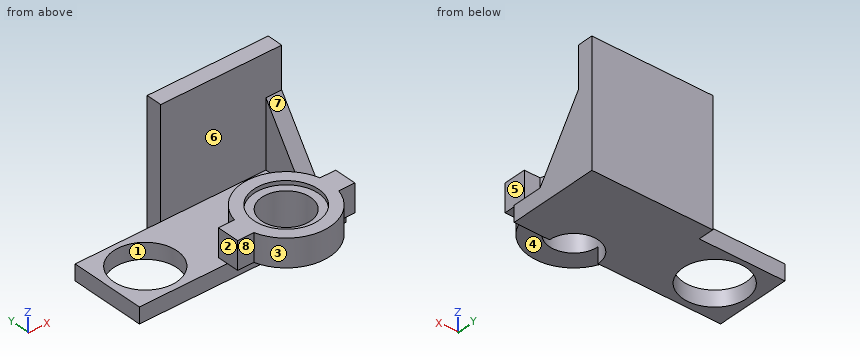
```python
from build123d import *

# Parameters (mm, degrees)
F0_W      = 52.233020775
F0_H      = 18.9497452229
F1_DEPTH  = 4
F2_D      = 16
F4_DEPTH  = 7
F5_R      = 6.15
F6_DEPTH  = 10
F7_R      = 8.15
F8_DEPTH  = 3.72
F9_W      = 30.5920690298
F9_H      = 31.4969494939
F10_DEPTH = 4
F12_DEPTH = 4


with BuildPart() as f1:
    # F0 (on Top) → F1 (new body)
    with BuildSketch(Plane.XY):
        with Locations((-11.0083804466, 9.4748726115)):
            Rectangle(F0_W, F0_H)
    extrude(amount=F1_DEPTH)

    # F2 (through all)
    with Locations(Plane(origin=(0, 0, 0), x_dir=(1, 0, 0), z_dir=(0, 0, -1))):
        with Locations((-27.3946430534, -9.6157854423)):
            Hole(F2_D / 2)

    # F3 (on face) → F4 (join)
    with BuildSketch(Plane.XY.offset(4)):
        with BuildLine():
            Line((-10.8105310121, 2.6503070258), (-14.8572139442, 2.6503070258))
            Line((-14.8572139442, 2.6503070258), (-14.8572139442, -3.0028291512))
            Line((-14.8572139442, -3.0028291512), (-10.7179627347, -3.0028291512))
            ThreePointArc((-10.7179627347, -3.0028291512), (-11.1291732807, -0.1822366147), (-10.8105310121, 2.6503070258))
        make_face()
        with BuildLine():
            ThreePointArc((10.8105310121, 2.6503070258), (0, 11.1306652135), (-10.8105310121, 2.6503070258))
            ThreePointArc((-10.8105310121, 2.6503070258), (-11.1291732807, -0.1822366147), (-10.7179627347, -3.0028291512))
            ThreePointArc((-10.7179627347, -3.0028291512), (0, -11.1306652135), (10.7179627347, -3.0028291512))
            ThreePointArc((10.7179627347, -3.0028291512), (11.1291732807, -0.1822366147), (10.8105310121, 2.6503070258))
        make_face()
        with BuildLine():
            Line((14.7918676957, 2.6503070258), (10.8105310121, 2.6503070258))
            ThreePointArc((10.8105310121, 2.6503070258), (11.1291732807, -0.1822366147), (10.7179627347, -3.0028291512))
            Line((10.7179627347, -3.0028291512), (14.7918676957, -3.0028291512))
            Line((14.7918676957, -3.0028291512), (14.7918676957, 2.6503070258))
        make_face()
    extrude(amount=F4_DEPTH)

    # F5 (on Top) → F6 (cut)
    with BuildSketch(Plane.XY):
        Circle(F5_R)
    extrude(amount=F6_DEPTH, mode=Mode.SUBTRACT)

    # F7 (on face) → F8 (cut)
    with BuildSketch(Plane(origin=(0, 0, 10), x_dir=(1, 0, 0), z_dir=(0, 0, -1))):
        Circle(F7_R)
    extrude(amount=-F8_DEPTH, mode=Mode.SUBTRACT)

    # F9 (on face) → F10 (join)
    with BuildSketch(Plane(origin=(0, 18.9497452229, 0), x_dir=(-1, 0, 0), z_dir=(0, 1, 0))):
        with Locations((0.187904574, 15.7484747469)):
            Rectangle(F9_W, F9_H)
    extrude(amount=F10_DEPTH)

    # F11 (on face) → F12 (join)
    with BuildSketch(Plane.YZ.offset(15.1081299409)):
        Polygon((18.9497452229, 20.9649894387), (7.6817818917, 4), (18.9497452229, 4), align=None)
    extrude(amount=-F12_DEPTH)


solid = f1.part
```
For this review, take the finished solid that the model builds, in its own axes (mm). Face numbers are marked on the shaded views. A direction names the side the tool comes from. Coordinates: 2 decimals unless noted, no trailing zeros. Write each loop counter-clockwise with the first axis right and the second up, starting at its lowest first coordinate (ties: lowest second). Pieces come first, ordered by that corner, then holes. Notation, with made-up numbers: (83, -30.75) -> (132, -30.75) arc R11 cw to (132, -22.75) -> close; hole circle Ø3 at (32.5, -8.5). An arc over 180 degrees is marked (long way). Put each result on its own line as item: value.
Q1. Take a section at A-A, the plane x = 0. State the section outline as (y, z) points, then the cut area to 3 significant figures.
From the geometry:
outline: (-11.13, 4) -> (-6.15, 4) -> (-6.15, 10) -> (-8.15, 10) -> (-8.15, 11) -> (-11.13, 11) -> close; (6.15, 0) -> (22.95, 0) -> (22.95, 31.5) -> (18.95, 31.5) -> (18.95, 4) -> (11.13, 4) -> (11.13, 11) -> (8.15, 11) -> (8.15, 10) -> (6.15, 10) -> close
area: 243 mm2
Q2. The part is to be moulded in two halves that separate along Y. For the marked faces 1, 2 and 3, say which applies: +Y half, -Y half, draft (parallel to the pull), parting line (faces both ways), or undercut.
From the geometry:
face 1: undercut
face 2: draft
face 3: -Y half
Q3. Clearance check with flat-ended pins moving along their axes: pin 1 Ø3.5 at (y, z) = (13.5, 14) entering from -X; pin 2 Ø1.7 at (y, z) = (0.5, 7.5) entering from +X; pin 3 Ø18 at (x, y) = (4, 3.5) entering from +Z; pin 4 Ø14.5 at (x, y) = (0, 0) entering from -Z. State where each tip first meets the part, or that it passes through.
From the geometry:
pin 1: stops at x = 11.11
pin 2: stops at x = 14.79
pin 3: stops at z = 11
pin 4: stops at z = 0
Q4. Take a section at D-D, the plane x = -28.5. State the section outline as (y, z) points.
From the geometry:
outline: (0, 0) -> (1.69, 0) -> (1.69, 4) -> (0, 4) -> close; (17.54, 0) -> (18.95, 0) -> (18.95, 4) -> (17.54, 4) -> close
Q5. Take a section at C-C, the plane y = 5. State the section outline as (x, z) points.
From the geometry:
outline: (-37.12, 0) -> (-33.93, 0) -> (-33.93, 4) -> (-37.12, 4) -> close; (-20.86, 0) -> (-3.58, 0) -> (-3.58, 10) -> (-6.44, 10) -> (-6.44, 11) -> (-9.94, 11) -> (-9.94, 4) -> (-20.86, 4) -> close; (3.58, 0) -> (15.11, 0) -> (15.11, 4) -> (9.94, 4) -> (9.94, 11) -> (6.44, 11) -> (6.44, 10) -> (3.58, 10) -> close
Q6. Tool access review of the marked faces 4, 5, 6, 7 and 8: name each direction out of +Z, -Z, +X, -X, +Y, -Y from which nothing blocks a thin tool from reaching the whole face with its end or side.
From the geometry:
face 4: -Z, +X, -X, -Y
face 5: +Z, +X, -Y
face 6: +Z, -X
face 7: +Z, +X
face 8: +Z, -Z, -X, -Y
Q7. Take a section at B-B, the plane y = -4. State the section outline as (x, z) points, then the cut area to 3 significant figures.
From the geometry:
outline: (-10.39, 4) -> (-4.67, 4) -> (-4.67, 10) -> (-7.1, 10) -> (-7.1, 11) -> (-10.39, 11) -> close; (4.67, 4) -> (10.39, 4) -> (10.39, 11) -> (7.1, 11) -> (7.1, 10) -> (4.67, 10) -> close
area: 75.2 mm2
Q8. Wall thickness on L1, parallel to Y at x = 0, z = 4.75; L2, parallel to Y at x = 0, z = 10.25; L3, parallel to Z at x = 11, y = -1.5: over which ranges is each line inside the solid? List them lowest first.
From the geometry:
L1: y = -11.13 to -6.15, 6.15 to 11.13, 18.95 to 22.95
L2: y = -11.13 to -8.15, 8.15 to 11.13, 18.95 to 22.95
L3: z = 4 to 11
